from build123d import *

# Parameters (mm, degrees)
F0_R     = 2.5
F1_DEPTH = 5


with BuildPart() as f1:
    # F0 (on Top) → F1 (new body)
    with BuildSketch(Plane.XY):
        with BuildLine():
            Line((-5, 15), (-12.5, 15))
            ThreePointArc((-12.5, 15), (-28.9528470752, 26.8585412256), (-35, 7.5))
            ThreePointArc((-35, 7.5), (-32.5, 0), (-35, -7.5))
            ThreePointArc((-35, -7.5), (-28.9528470752, -26.8585412256), (-12.5, -15))
            Line((-12.5, -15), (12.6964542654, -15))
            ThreePointArc((12.6964542654, -15), (29.1493013406, -26.8585412256), (35.1964542654, -7.5))
            ThreePointArc((35.1964542654, -7.5), (32.784838444, 0.0710641767), (35.1964542654, 7.6421283534))
            ThreePointArc((35.1964542654, 7.6421283534), (28.8541630659, 26.7626213853), (12.5, 15))
            Line((12.5, 15), (5, 15))
            ThreePointArc((5, 15), (0, 20), (-5, 15))
        make_face()
        with BuildLine():
            add(Edge.make_bspline(
                [(-14.9199757765, -0.4431015054), (-14.4528073363, -0.9517960291), (-14.4528073363, -1.7615546588)],
                knots=[0, 0, 0, 1, 1, 1], degree=2))
            add(Edge.make_bspline(
                [(-14.4528073363, -1.7615546588), (-14.4528073363, -2.8048975085), (-15.2097932347, -3.3897231855)],
                knots=[0, 0, 0, 1, 1, 1], degree=2))
            add(Edge.make_bspline(
                [(-15.2097932347, -3.3897231855), (-15.9667791331, -3.9745488624), (-17.2644692447, -3.9745488624)],
                knots=[0, 0, 0, 1, 1, 1], degree=2))
            add(Edge.make_bspline(
                [(-17.2644692447, -3.9745488624), (-18.6694350722, -3.9745488624), (-19.4272860974, -3.6111956312)],
                knots=[0, 0, 0, 1, 1, 1], degree=2))
            Line((-19.4272860974, -3.6111956312), (-19.4272860974, -2.7253058483))
            add(Edge.make_bspline(
                [(-19.4272860974, -2.7253058483), (-18.9393546155, -2.9294757592), (-18.3666407129, -3.0488632495)],
                knots=[0, 0, 0, 1, 1, 1], degree=2))
            add(Edge.make_bspline(
                [(-18.3666407129, -3.0488632495), (-17.7939268103, -3.1682507397), (-17.2315944286, -3.1682507397)],
                knots=[0, 0, 0, 1, 1, 1], degree=2))
            add(Edge.make_bspline(
                [(-17.2315944286, -3.1682507397), (-16.3128298296, -3.1682507397), (-15.8473916429, -2.8196046631)],
                knots=[0, 0, 0, 1, 1, 1], degree=2))
            add(Edge.make_bspline(
                [(-15.8473916429, -2.8196046631), (-15.3819534562, -2.4709585864), (-15.3819534562, -1.8480673329)],
                knots=[0, 0, 0, 1, 1, 1], degree=2))
            add(Edge.make_bspline(
                [(-15.3819534562, -1.8480673329), (-15.3819534562, -1.4379972576), (-15.5471926637, -1.1758638551)],
                knots=[0, 0, 0, 1, 1, 1], degree=2))
            add(Edge.make_bspline(
                [(-15.5471926637, -1.1758638551), (-15.7124318713, -0.9137304525), (-16.0991435245, -0.6913928801)],
                knots=[0, 0, 0, 1, 1, 1], degree=2))
            add(Edge.make_bspline(
                [(-16.0991435245, -0.6913928801), (-16.4858551778, -0.4690553076), (-17.2748507656, -0.1887542435)],
                knots=[0, 0, 0, 1, 1, 1], degree=2))
            add(Edge.make_bspline(
                [(-17.2748507656, -0.1887542435), (-18.3770222338, 0.2057435504), (-18.8502465611, 0.7464477636)],
                knots=[0, 0, 0, 1, 1, 1], degree=2))
            add(Edge.make_bspline(
                [(-18.8502465611, 0.7464477636), (-19.3234708885, 1.2871519767), (-19.3234708885, 2.1574694783)],
                knots=[0, 0, 0, 1, 1, 1], degree=2))
            add(Edge.make_bspline(
                [(-19.3234708885, 2.1574694783), (-19.3234708885, 3.0710433168), (-18.6374253828, 3.61174753)],
                knots=[0, 0, 0, 1, 1, 1], degree=2))
            add(Edge.make_bspline(
                [(-18.6374253828, 3.61174753), (-17.9513798772, 4.1524517432), (-16.8197940998, 4.1524517432)],
                knots=[0, 0, 0, 1, 1, 1], degree=2))
            add(Edge.make_bspline(
                [(-16.8197940998, 4.1524517432), (-15.6414914785, 4.1524517432), (-14.6517864867, 3.7198883726)],
                knots=[0, 0, 0, 1, 1, 1], degree=2))
            Line((-14.6517864867, 3.7198883726), (-14.9390085648, 2.9205112639))
            add(Edge.make_bspline(
                [(-14.9390085648, 2.9205112639), (-15.9183320356, 3.3305813392), (-16.8422873951, 3.3305813392)],
                knots=[0, 0, 0, 1, 1, 1], degree=2))
            add(Edge.make_bspline(
                [(-16.8422873951, 3.3305813392), (-17.5724543646, 3.3305813392), (-17.9833895666, 3.0174054589)],
                knots=[0, 0, 0, 1, 1, 1], degree=2))
            add(Edge.make_bspline(
                [(-17.9833895666, 3.0174054589), (-18.3943247686, 2.7042295786), (-18.3943247686, 2.1470879574)],
                knots=[0, 0, 0, 1, 1, 1], degree=2))
            add(Edge.make_bspline(
                [(-18.3943247686, 2.1470879574), (-18.3943247686, 1.7370178821), (-18.2429275889, 1.4740193528)],
                knots=[0, 0, 0, 1, 1, 1], degree=2))
            add(Edge.make_bspline(
                [(-18.2429275889, 1.4740193528), (-18.0915304092, 1.2110208235), (-17.7316376849, 0.992143758)],
                knots=[0, 0, 0, 1, 1, 1], degree=2))
            add(Edge.make_bspline(
                [(-17.7316376849, 0.992143758), (-17.3717449606, 0.7732666926), (-16.6311964703, 0.5085379098)],
                knots=[0, 0, 0, 1, 1, 1], degree=2))
            add(Edge.make_bspline(
                [(-16.6311964703, 0.5085379098), (-15.3871442166, 0.0655930184), (-14.9199757765, -0.4431015054)],
                knots=[0, 0, 0, 1, 1, 1], degree=2))
        make_face(mode=Mode.SUBTRACT)
        Polygon((-6.9140929146, -3.865542893), (-7.8657323298, -3.865542893), (-8.8502465611, -1.3514845835), (-12.0183406869, -1.3514845835), (-12.9907431439, -3.865542893), (-13.9216195173, -3.865542893), (-10.7967817285, 4.072860083), (-10.023358422, 4.072860083), align=None, mode=Mode.SUBTRACT)
        with BuildLine():
            Line((-1.5883726966, -3.865542893), (-2.328921187, -3.865542893))
            Line((-2.328921187, -3.865542893), (-5.0108140843, 3.1419837096))
            Line((-5.0108140843, 3.1419837096), (-5.0540704213, 3.1419837096))
            add(Edge.make_bspline(
                [(-5.0540704213, 3.1419837096), (-4.9779392681, 2.3097317847), (-4.9779392681, 1.162573726)],
                knots=[0, 0, 0, 1, 1, 1], degree=2))
            Line((-4.9779392681, 1.162573726), (-4.9779392681, -3.865542893))
            Line((-4.9779392681, -3.865542893), (-5.8274937278, -3.865542893))
            Line((-5.8274937278, -3.865542893), (-5.8274937278, 4.0399852668))
            Line((-5.8274937278, 4.0399852668), (-4.4432909421, 4.0399852668))
            Line((-4.4432909421, 4.0399852668), (-1.9396141535, -2.4813401073))
            Line((-1.9396141535, -2.4813401073), (-1.8963578164, -2.4813401073))
            Line((-1.8963578164, -2.4813401073), (0.628082014, 4.0399852668))
            Line((0.628082014, 4.0399852668), (2.0019032788, 4.0399852668))
            Line((2.0019032788, 4.0399852668), (2.0019032788, -3.865542893))
            Line((2.0019032788, -3.865542893), (1.0831386798, -3.865542893))
            Line((1.0831386798, -3.865542893), (1.0831386798, 1.2283233584))
            add(Edge.make_bspline(
                [(1.0831386798, 1.2283233584), (1.0831386798, 2.1038316203), (1.159269833, 3.1316021887)],
                knots=[0, 0, 0, 1, 1, 1], degree=2))
            Line((1.159269833, 3.1316021887), (1.116013496, 3.1316021887))
            Line((1.116013496, 3.1316021887), (-1.5883726966, -3.865542893))
        make_face(mode=Mode.SUBTRACT)
        with Locations((0, 15)):
            Circle(F0_R, mode=Mode.SUBTRACT)
        with BuildLine():
            Line((8.4090319232, -3.865542893), (7.6684834328, -3.865542893))
            Line((7.6684834328, -3.865542893), (4.9865905355, 3.1419837096))
            Line((4.9865905355, 3.1419837096), (4.9433341985, 3.1419837096))
            add(Edge.make_bspline(
                [(4.9433341985, 3.1419837096), (5.0194653517, 2.3097317847), (5.0194653517, 1.162573726)],
                knots=[0, 0, 0, 1, 1, 1], degree=2))
            Line((5.0194653517, 1.162573726), (5.0194653517, -3.865542893))
            Line((5.0194653517, -3.865542893), (4.1699108919, -3.865542893))
            Line((4.1699108919, -3.865542893), (4.1699108919, 4.0399852668))
            Line((4.1699108919, 4.0399852668), (5.5541136777, 4.0399852668))
            Line((5.5541136777, 4.0399852668), (8.0577904663, -2.4813401073))
            Line((8.0577904663, -2.4813401073), (8.1010468034, -2.4813401073))
            Line((8.1010468034, -2.4813401073), (10.6254866338, 4.0399852668))
            Line((10.6254866338, 4.0399852668), (11.9993078986, 4.0399852668))
            Line((11.9993078986, 4.0399852668), (11.9993078986, -3.865542893))
            Line((11.9993078986, -3.865542893), (11.0805432996, -3.865542893))
            Line((11.0805432996, -3.865542893), (11.0805432996, 1.2283233584))
            add(Edge.make_bspline(
                [(11.0805432996, 1.2283233584), (11.0805432996, 2.1038316203), (11.1566744528, 3.1316021887)],
                knots=[0, 0, 0, 1, 1, 1], degree=2))
            Line((11.1566744528, 3.1316021887), (11.1134181158, 3.1316021887))
            Line((11.1134181158, 3.1316021887), (8.4090319232, -3.865542893))
        make_face(mode=Mode.SUBTRACT)
        Polygon((14.0859935981, 4.0399852668), (16.1796003114, 0.0863560601), (18.2870490527, 4.0399852668), (19.2819448049, 4.0399852668), (16.6433082447, -0.7995337227), (16.6433082447, -3.865542893), (15.7141621248, -3.865542893), (15.7141621248, -0.8427900598), (13.0807163249, 4.0399852668), align=None, mode=Mode.SUBTRACT)
    extrude(amount=F1_DEPTH)


solid = f1.part
CAD build for the part. Positions are in the model's coordinates, mm. A direction names the side the tool comes from. Give positions to 0.01 mm unless a question says otherwise; leave off trailing zeros. Write each loop counter-clockwise with the first axis right and the second up, starting at its lowest first coordinate (ties: lowest second). Pieces come first, ordered by that corner, then holes. Notation, with made-up numbers: M -36.5,6 L -3.5,6 A7 ccw -3.5,13 Z; hole C -38,-2 d4. An arc over 180 degrees is marked long. Put each result on its own line as item: value. Start each with the question number.
(1) Which spindle directions (+Z, -Z, +X, -X, +Y, -Y) get a long thin tool onto all of the face, cutting with end or side? Do faces 4 (the face through (32.785, -0.042, 2.465)), 5 (the face through (9, 15, 2)), 6 (the face through (-0.652, 0.734, 2.465)). Say none if no direction does.
(2) Mould opens along Y. For faces 1 (the face through (0, 20, 2)), 2 (the face through (0, -15, 2)), 3 (the face through (9.346, 0.734, 2.465)) say: +Y half, -Y half, draft (parallel to the pull), parting line (faces both ways), or undercut.
(3) Band-saw the part on B-B, the plane z = 2.1. Give the number of separate pieces and of enclosed holes in the cut face, and give its area (3 significant figures).
(4) Band-saw the part on D-D, the plane y = -9.5. Write the cut outline in (x, z).
(5) Band-saw the part on A-A, the plane y = -16. Write the cut outline in (x, z).
(6) Flat gauge pins, fed straight in: pin 1 Ø12 at (x, y) = (-10.5, 5.5) entering from -Z; pin 2 Ø0.8 at (x, z) = (13.5, 1.5) entering from -Y; pin 3 Ø1.1 at (x, z) = (19, 2.5) entering from -Y; pin 4 Ø0.8 at (x, z) = (-2, 3) entering from +Y. Where does each tip first touch, or does it go through?
(7) Band-saw the part on C-C, the plane y = 6. Write the cut outline in (x, z), and give its area (3 significant figures).
(8) Probe L1, parallel to X at y = -7.5, z = 1.4; L2, parallel to X at y = -25, z = 0.9; L3, parallel to X at y = 24, z = 0.5. List the from-to ranges inside material, lowest first.
Response values:
1. face 4: +Z, -Z, +X
1. face 5: +Z, -Z, +Y
1. face 6: +Z, -Z
2. face 1: +Y half
2. face 2: -Y half
2. face 3: undercut
3. separate pieces: 1
3. enclosed holes: 6
3. area: 3,000 mm2
4. outline: M -36.22,0 L 36.42,0 L 36.42,5 L -36.22,5 Z
5. outline: M -37.46,0 L -12.54,0 L -12.54,5 L -37.46,5 Z; M 12.74,0 L 37.66,0 L 37.66,5 L 12.74,5 Z
6. pin 1: stops at z = 0
6. pin 2: stops at y = -20.35
6. pin 3: stops at y = -26.15
6. pin 4: stops at y = 19.74
7. outline: M -34.03,0 L 34.2,0 L 34.2,5 L -34.03,5 Z
7. area: 341 mm2
8. L1: x = -35 to 35.2
8. L2: x = -32.5 to -17.5, 17.7 to 32.7
8. L3: x = -33.67 to -16.33, 16.46 to 33.54
